Here's how the part is built. I have some questions about the finished solid (model axes, mm). A direction names the side the tool comes from. Give positions to 0.01 mm unless a question says otherwise; leave off trailing zeros. Loops run counter-clockwise (first coordinate to the right, second up) from the corner with the lowest first, then second, coordinate; pieces in that order, holes last. Notation, with made-up numbers: M -14.5,-24.75 L -3.5,-24.75 A35 ccw -3.5,9.25 Z; hole C -16.5,67 d5. An arc over 180 degrees is marked long. Write item = value, one per line. Start each with the question number.
```python
from build123d import *

# Parameters (mm, degrees)
F0_W     = 6.35
F0_H     = 33.401
F2_R     = 1.524
F3_W     = 5.08
F3_H     = 28.219457
F4_DEPTH = 12.7
F5_R     = 0.762


with BuildPart() as f1:
    # F0 (on Front) → F1 (revolve)
    with BuildSketch(Plane.XZ):
        with Locations((3.175, 16.7005)):
            Rectangle(F0_W, F0_H)
    revolve(axis=Axis((0, 0, 16.7005), (0, 0, 1)))

    # F2
    f2_edges = [f1.edges().sort_by_distance(p)[0] for p in [
        (-6.35, 0, 0),
        (-6.35, 0, 33.401),
        (6.35, 0, 16.7005),
    ]]
    fillet(f2_edges, radius=F2_R)

    # F3 (on Front) → F4 (cut, symmetric)
    with BuildSketch(Plane.XZ):
        with Locations((6.35, 20.459729)):
            Rectangle(F3_W, F3_H)
    extrude(amount=F4_DEPTH, both=True, mode=Mode.SUBTRACT)

    # F5
    f5_edges = [f1.edges().sort_by_distance(p)[0] for p in [
        (5.679613, 2.839806, 6.35),
        (5.679613, -2.839806, 6.35),
    ]]
    fillet(f5_edges, radius=F5_R)


solid = f1.part
```
Q1. Will these pins go through, and if not, where does the flat tip stop? pin 1 (3 mm diameter, centred on y = 2, z = 26, fed in from +X); pin 2 (3 mm diameter, centred on x = 5, y = -4.5, fed in from -Z); pin 3 (3 mm diameter, centred on x = 2.5, z = 20, fed in from -Y).
Q2. If I drill on line 1 along X through (y, z) = (0.25, 3); line 2 along Z through (x, y) = (-0.5, -5); line 3 along Y through (x, z) = (-3.25, 7), over which ranges is the centre line in solid material (lowest first)?
Q3. If we section it at A-A, the plane y = 0: List the corners of the cut face in (x, z) for me, then the cut area to 3 significant figures.
Q4. On a 3-axis mill with a long thin cutter (end or side, diameter ignored), from which of +Z, -Z, +X, -X, +Y, -Y can I reach the whole of each face in a straight line? I mean faces 1 (the flat face through (4, 0, 6.35)), 2 (the cylindrical face through (-6.344, 0.279, 16.913)). Say none if no direction works.
Q5. If we section it at B-B, the plane z = 10: List the corners of the cut face in (x, y) for me, then the cut area to 3 significant figures.
Resolved:
q1.pin_1 = 3.81
q1.pin_2 = 0.05
q1.pin_3 = -6.27
q2.line_1 = -6.35 to 6.35
q2.line_2 = 0.01 to 33.39
q2.line_3 = -5.46 to 5.46
q3.outline = M -6.35,1.52 A1.52 ccw -4.83,0 L 4.83,0 A1.52 ccw 6.35,1.52 L 6.35,5.59 A0.76 ccw 5.59,6.35 L 3.81,6.35 L 3.81,33.4 L -4.83,33.4 A1.52 ccw -6.35,31.88 Z
q3.area = 354 mm²
q4.face_1 = +Z, +X, +Y, -Y
q4.face_2 = +Z, -Z
q5.outline = M 3.81,-5.08 L 3.81,5.08 A6.35 ccw long Z
q5.area = 109 mm²
